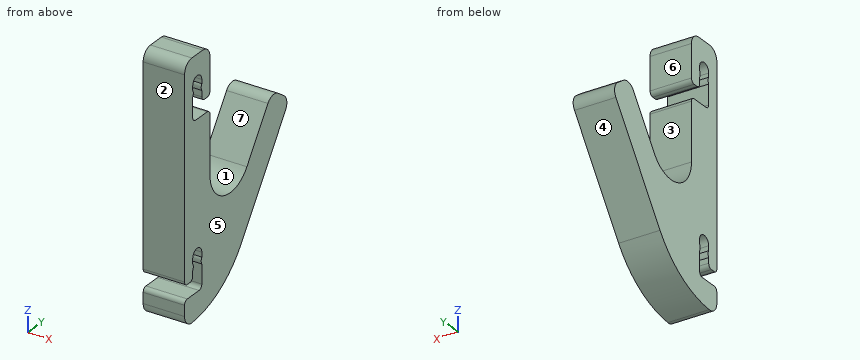
from build123d import *

# Parameters (mm, degrees)
F1_DEPTH = 3.81
F2_R     = 2.032
F4_DEPTH = 7.621
F5_R     = 0.762
F7_DEPTH = 7.62


# Not quite as in the source:
# - a feature names something its author has since deleted; it is built from what else it names


with BuildPart() as f1:
    # F0 (on Right) → F1 (new body, symmetric)
    with BuildSketch(Plane.YZ):
        with BuildLine():
            Line((0, 42.3580370843), (0, 0))
            Line((0, 0), (0, -3.979871033))
            ThreePointArc((0, -3.979871033), (8.9499402185, -2.2460183558), (15.9004898533, 3.6529251764))
            Line((15.9004898533, 3.6529251764), (29.4239599312, 22.9664420122))
            Line((29.4239599312, 22.9664420122), (24.5073227445, 26.4091084329))
            Line((24.5073227445, 26.4091084329), (17.4524241549, 16.3336690744))
            ThreePointArc((17.4524241549, 16.3336690744), (11.0805919315, 14.1707234894), (7.1017071605, 19.5972376068))
            Line((7.1017071605, 19.5972376068), (7.1017071605, 42.3580370843))
            Line((7.1017071605, 42.3580370843), (0, 42.3580370843))
        make_face()
    extrude(amount=F1_DEPTH, both=True)

    # F2
    f2_edges = [f1.edges().sort_by_distance(p)[0] for p in [
        (0, 7.101707, 42.358037),
        (0, 0, 42.358037),
        (0, 29.42396, 22.966442),
        (0, 24.507323, 26.409108),
        (0, 0, -3.979871),
    ]]
    fillet(f2_edges, radius=F2_R)

    # F3 (on face) → F4 (cut, through all)
    with BuildSketch(Plane.YZ.offset(3.81)):
        with BuildLine():
            Line((4.8208535802, 33.5311107337), (4.8208535802, 37.3411107337))
            ThreePointArc((4.8208535802, 37.3411107337), (3.5508535802, 38.6111107337), (2.2808535802, 37.3411107337))
            Line((2.2808535802, 37.3411107337), (2.2808535802, 30.9911107337))
            Line((2.2808535802, 30.9911107337), (7.1017071605, 30.9911107337))
            Line((7.1017071605, 30.9911107337), (7.1017071605, 33.5311107337))
            Line((7.1017071605, 33.5311107337), (4.8208535802, 33.5311107337))
        make_face()
        with BuildLine():
            Line((4.8208535802, 0.7651107337), (4.8208535802, 7.1151107337))
            ThreePointArc((4.8208535802, 7.1151107337), (3.5508535802, 8.3851107337), (2.2808535802, 7.1151107337))
            Line((2.2808535802, 7.1151107337), (2.2808535802, 3.3051107337))
            Line((2.2808535802, 3.3051107337), (0, 3.3051107337))
            Line((0, 3.3051107337), (0, 0.7651107337))
            Line((0, 0.7651107337), (4.8208535802, 0.7651107337))
        make_face()
    extrude(amount=-F4_DEPTH, mode=Mode.SUBTRACT)

    # F5
    f5_edges = [f1.edges().sort_by_distance(p)[0] for p in [
        (0, 4.820854, 33.531111),
        (0, 7.101707, 33.531111),
        (0, 2.280854, 30.991111),
        (0, 7.101707, 30.991111),
        (0, 0, 3.305111),
        (0, 4.820854, 0.765111),
        (0, 0, 0.765111),
        (0, 2.280854, 3.305111),
    ]]
    fillet(f5_edges, radius=F5_R)

    # F6 (on face) → F7 (join, through all)
    with BuildSketch(Plane.YZ.offset(3.81)):
        with BuildLine():
            Line((4.8208535802, 35.4121252894), (4.8208535802, 36.6062968969))
            ThreePointArc((4.8208535802, 36.6062968969), (4.6525009744, 36.0092110932), (4.8208535802, 35.4121252894))
        make_face()
        with BuildLine():
            Line((2.2808535802, 36.6062968969), (2.2808535802, 35.4121252894))
            ThreePointArc((2.2808535802, 35.4121252894), (2.4492061861, 36.0092110932), (2.2808535802, 36.6062968969))
        make_face()
        with BuildLine():
            Line((2.2808535802, 6.2474817969), (2.2808535802, 5.0533101894))
            ThreePointArc((2.2808535802, 5.0533101894), (2.4492061861, 5.6503959931), (2.2808535802, 6.2474817969))
        make_face()
        with BuildLine():
            ThreePointArc((4.8208535802, 6.2474817969), (4.6525009744, 5.6503959931), (4.8208535802, 5.0533101894))
            Line((4.8208535802, 5.0533101894), (4.8208535802, 6.2474817969))
        make_face()
    extrude(amount=-F7_DEPTH)


solid = f1.part
Build history of the part. All positions in model axes, mm. Face numbers are marked on the shaded views. A direction names the side the tool comes from. Coordinates: 2 decimals unless noted, no trailing zeros. Order: outer loops, then holes, each group sorted by start corner. A loop starts at its lowest first (then second) coordinate and runs counter-clockwise, first axis right, second up. Notation, with made-up numbers: (73.25, 35.5) -> (98.25, 35.5) arc R16 ccw to (98.25, 45.5) -> close; hole circle Ø2 at (51.5, 73). An arc over 180 degrees is marked (long way). One line per item, written item: value.
(1) Drop flat-ended pins along their axis: pin 1 Ø1.1 at (x, z) = (2, 3) entering from -Y; pin 2 Ø0.6 at (x, y) = (1.5, 6) entering from -Z; pin 3 Ø1.8 at (x, z) = (-2, 33.5) entering from +Y. Give the stop position or say it passes through.
Checked values:
pin 1: y = 0.2
pin 2: z = -3.44
pin 3: y = 7.1
(2) Mould opens along Y. For the marked faces 1, 2, 3 and 4 say: pulls with the +Y half, pulls with the -Y half, needs draft (parallel to the pull), parting line crosses it, or undercut.
Checked values:
face 1: undercut
face 2: pulls with the -Y half
face 3: undercut
face 4: pulls with the +Y half
(3) Slice it at A-A, the plane z = 39.5. List the corners of the cut face in (x, y), plus the area to 3 significant figures.
Checked values:
outline: (-3.81, 0) -> (3.81, 0) -> (3.81, 7.1) -> (-3.81, 7.1) -> close
area: 54.1 mm2
(4) Tool access for the marked faces 5, 6 and 7: list every direction of +Z, -Z, +X, -X, +Y, -Y with a clear straight run to the whole face (end or side of a thin tool).
Checked values:
face 5: +Z, -Z, +X, +Y, -Y
face 6: +Z, +X, -X, +Y
face 7: +Z, +X, -X
(5) Probe line 1 (Y direction, x = -0.5, z = 20); line 2 (Z direction, x = -1, y = 5); line 3 (Y direction, x = 0.75, z = 16.5). List the from-to ranges inside material, lowest first. Write a range as [from, to].
Checked values:
line 1: [0, 7.1], [20.02, 27.35]
line 2: [-3.6, 30.99], [33.8, 42.36]
line 3: [0, 8.02], [17.57, 24.9]
(6) Slice it at B-B, the plane y = 26.75. List the corners of the cut face in (x, z), plus the area to 3 significant figures.
Checked values:
outline: (-3.81, 19.15) -> (3.81, 19.15) -> (3.81, 24.84) -> (-3.81, 24.84) -> close
area: 43.4 mm2
